```python
from build123d import *

# Parameters (mm, degrees)
SKETCH1_R               = 2.25
BOSS_EXTRUDE1_DEPTH     = 180
FILLET1_R               = 0.75
SKETCH2_R               = 1.1
CUT_EXTRUDE1_DEPTH      = 3.25
CUT_EXTRUDE1_DEPTH_BACK = 3.25


with BuildPart() as part:
    # Sketch1 → Boss-Extrude1 (new body)
    with BuildSketch(Plane(origin=(0, 0, 0), x_dir=(0, 0, -1), z_dir=(1, 0, 0))):
        Circle(SKETCH1_R)
    extrude(amount=BOSS_EXTRUDE1_DEPTH)

    # Fillet1
    fillet1_edges = [part.edges().sort_by_distance(p)[0] for p in [
        (0, 0, 2.25),
    ]]
    fillet(fillet1_edges, radius=FILLET1_R)

    # Sketch2 → Cut-Extrude1 (cut, two sides)
    with BuildSketch(Plane.XY) as cut_extrude1_sk:
        with BuildLine():
            Line((180, 2.25), (177.75, 2.25))
            ThreePointArc((177.75, 2.25), (179.340990258, 1.590990258), (180, 0))
            Line((180, 0), (180, 2.25))
        make_face()
        with BuildLine():
            Line((180, -2.25), (180, 0))
            ThreePointArc((180, 0), (179.340990258, -1.590990258), (177.75, -2.25))
            Line((177.75, -2.25), (180, -2.25))
        make_face()
        with Locations((177.75, 0)):
            Circle(SKETCH2_R)
    extrude(amount=CUT_EXTRUDE1_DEPTH, mode=Mode.SUBTRACT)
    extrude(cut_extrude1_sk.sketch, amount=-CUT_EXTRUDE1_DEPTH_BACK, mode=Mode.SUBTRACT)


solid = part.part
```
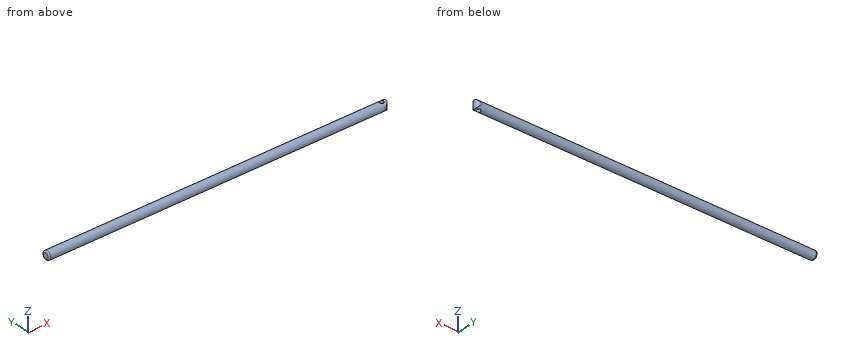
Part model, mm, in its own coordinate system. Coordinates: 2 decimals unless noted, no trailing zeros. Order: outer loops, then holes, each group sorted by start corner. A loop starts at its lowest first (then second) coordinate and runs counter-clockwise, first axis right, second up. Notation, with made-up numbers: (88, -2) - (94, -2) arc R19 cw to (94, 31) - close; hole circle Ø6 at (81.5, -5). An arc over 180 degrees is marked (long way). Return JSON: item names as keys, results as strings. Group by question number.
Item 1: Cut at A-A (x = 87.5). List the corners of the cut face in (y, z).
Item 2: Pin check, flat tips, straight feed: pin 1 (2 mm diameter, centred on x = 177.75, y = 0, fed in from -Z); pin 2 (2 mm diameter, centred on x = 135, z = 1.5, fed in from -Y); pin 3 (1.5 mm diameter, centred on x = 149.5, y = 1.5, fed in from +Z). Stop position of each tip, or through.
Item 3: Drill centre lines: probe 1 along X at (y, z) = (0, 0.4); probe 2 along Y at (x, z) = (177.75, 0.25); probe 3 along Z at (x, y) = (68, -0.25). Where is each one in solid material? Low to high. Write a range as from..to.
Check values:
{
 "1": {"outline": "circle Ø4.5 at (0, 0)"},
 "2": {"pin 1": "passes through", "pin 2": "stops at y = -2.19", "pin 3": "stops at z = 2.12"},
 "3": {"probe 1": "x = 0..176.65, 178.85..180", "probe 2": "y = -2.24..-1.1, 1.1..2.24", "probe 3": "z = -2.24..2.24"}
}
